Autodesk Inventor part; units mm, degrees
ref_plane "YZ Plane" through (0, 0, 0) normal (1, 0, 0) x (0, 1, 0)
ref_plane "XZ Plane" through (0, 0, 0) normal (0, 1, 0) x (-1, 0, 0)
ref_plane "XY Plane" through (0, 0, 0) normal (0, 0, 1) x (1, 0, 0)
sketch "Sketch1" plane through (0, 0, 0) normal (0, 0, 1) x (1, 0, 0)
  line L0 (-50, -180) -> (-450, -180)
  line L1 (-450, -180) -> (-450, 120)
  line L2 (-450, 120) -> (-50, 120)
  line L3 (-50, 120) -> (-50, -180)
  point P0 (0, 0)
  dimension "d0" = 50
  dimension "d1" = 300
  dimension "d2" = 400
  dimension "d3" = 120
extrude "Extrusion1" add sketch "Sketch1" along normal blind 120
sketch "Sketch2" plane through (-450, 120, 0) normal (0, 1, 0) x (1, 0, 0)
  line L0 (0, 0) -> (400, 0)
  line L1 (0, 0) -> (0, -120)
  line L2 (0, -120) -> (400, -120)
  line L3 (400, 0) -> (400, -120)
  line L4 (205, -30) -> (180, -30)
  line L5 (180, -30) -> (180, -20)
  line L6 (180, -20) -> (205, -20)
  line L7 (205, -20) -> (205, -30)
  dimension "d6" = 25
  dimension "d7" = 10
  dimension "d8" = 20
  dimension "d9" = 220
extrude "Extrusion2" add sketch "Sketch2" along normal blind 10 contours L4 L5 L6 L7
pattern_linear "Rectangular Pattern1" count 4 spacing 50 along (-1, 0, 0) of "Extrusion2"
sketch "Sketch3" plane through (-450, 120, 0) normal (0, 1, 0) x (1, 0, 0)
  line L0 (0, -120) -> (400, -120)
  line L1 (400, 0) -> (400, -120)
  line L2 (0, 0) -> (400, 0)
  line L3 (0, 0) -> (0, -120)
  line L4 (15, -65) -> (300, -65)
  line L5 (300, -65) -> (300, -105)
  line L6 (300, -105) -> (15, -105)
  line L7 (15, -105) -> (15, -65)
  line L8 (330, -65) -> (345, -65)
  line L9 (345, -65) -> (345, -105)
  line L10 (345, -105) -> (330, -105)
  line L11 (330, -105) -> (330, -65)
  line L12 (360, -65) -> (375, -65)
  line L13 (375, -65) -> (375, -105)
  line L14 (375, -105) -> (360, -105)
  line L15 (360, -105) -> (360, -65)
  point P0 (450, 0)
  dimension "d15" = 65
  dimension "d16" = 15
  dimension "d17" = 15
  dimension "d18" = 100
  dimension "d21" = 30
  dimension "d22" = 15
  dimension "d23" = 15
extrude "Extrusion3" cut sketch "Sketch3" against normal blind 5 contours L4 L5 L6 L7 | L8 L9 L10 L11 | L12 L13 L14 L15
chamfer "Chamfer1" distance 4 angle 45 3 edges at (-450, -30, 120) (-450, -30, 0) (-50, -30, 0)
sketch "Sketch4" plane through (-446, 120, 0) normal (0, 1, 0) x (1, 0, 0)
  line L0 (392, 0) -> (396, -4)
  line L1 (0, 0) -> (392, 0)
  line L2 (-4, -4) -> (0, 0)
  line L3 (-4, -4) -> (-4, -116)
  line L4 (0, -120) -> (-4, -116)
  line L5 (0, -120) -> (396, -120)
  line L6 (396, -4) -> (396, -120)
  line L7 (389.8859, -5.1039) -> (390.8961, -6.1141)
  line L8 (390.8961, -6.1141) -> (390.8961, -114.8961)
  line L9 (390.8961, -114.8961) -> (2.1141, -114.8961)
  line L10 (2.1141, -114.8961) -> (1.1039, -113.8859)
  line L11 (1.1039, -113.8859) -> (1.1039, -6.1141)
  line L12 (1.1039, -6.1141) -> (2.1141, -5.1039)
  line L13 (2.1141, -5.1039) -> (389.8859, -5.1039)
  point P0 (446, 0)
extrude "Extrusion4" add sketch "Sketch4" along normal blind 2
properties part number "AbstractBox"
The listing builds one solid part. Answer for the finished solid, in the listing's coordinates (mm). A direction names the side the tool comes from. Coordinates: 2 decimals unless noted, no trailing zeros. Order: outer loops, then holes, each group sorted by start corner. A loop starts at its lowest first (then second) coordinate and runs counter-clockwise, first axis right, second up. Notation, with made-up numbers: M 53,-34 L 98,-34 A5 ccw 98,-26 Z; hole C 33,-23.5 d11. An arc over 180 degrees is marked long. Answer as a JSON object with one key per item and string values. Group by question number.
1. A tool of negligible diameter and unlimited length cuts with its end or side. For faces 4 (the flat face through (-50, -31, 61)), 5 (the flat face through (-345, 125, 25)), from which of +Z, -Z, +X, -X, +Y, -Y can it reach the whole face along a straight path? Write none if from no direction.
2. Section B-B on x = -140 is taken. Write down the section's boundary in (y, z).
3. Section D-D on z = 79.5 is taken. Write down the section's boundary in (x, y).
4. Straight lines are drawn through the part: line 1 (Y direction, x = -404.5, z = 49); line 2 (Y direction, x = -237, z = 96.5). For each, find the intervals that lie inside material, in ascending order.
5. Section C-C on x = -334.5 is taken. Write down the section's boundary in (y, z), then the cut area to 3 significant figures.
6. Section A-A on z = 40.5 is taken. Write down the section's boundary in (x, y).
7. Flat-ended cylindrical pins translate along their axes: P1, Ø5, axis at x = -351.5, y = 125.5, coming from the -Z side; P2, Ø5, axis at x = -358.5, y = 126.5, coming from the +Z side; P3, Ø10, axis at x = -156.5, z = 26.5, coming from the +Y side. Find the tip coordinate at first contact, or state that the pin passes through.
8. Determine the mould class of faces 1 (the flat face through (-251, -31, 120)), 2 (the flat face through (-295, 125, 25)), 3 (the flat face through (-450, -31, 59)) for opening direction Z: released by +Z, released by -Z, zero draft, split by the parting line, or undercut.
Values follow:
{
 "1": {"face 4": "+Z, -Z, +X, +Y, -Y", "face 5": "+Y"},
 "2": {"outline": "M -180,0 L 122,0 L 122,5.1 L 120,5.1 L 120,114.9 L 122,114.9 L 122,120 L -180,120 Z"},
 "3": {"outline": "M -450,-180 L -50,-180 L -50,122 L -55.1,122 L -55.1,120 L -75,120 L -75,115 L -90,115 L -90,120 L -105,120 L -105,115 L -120,115 L -120,120 L -150,120 L -150,115 L -435,115 L -435,120 L -444.9,120 L -444.9,122 L -450,122 Z"},
 "4": {"line 1": "-180 to 120", "line 2": "-180 to 115"},
 "5": {"outline": "M -180,0 L 122,0 L 122,5.1 L 120,5.1 L 120,65 L 115,65 L 115,105 L 120,105 L 120,114.9 L 122,114.9 L 122,120 L -180,120 Z", "area": "35,800 mm2"},
 "6": {"outline": "M -450,-180 L -50,-180 L -50,122 L -55.1,122 L -55.1,120 L -444.9,120 L -444.9,122 L -450,122 Z"},
 "7": {"P1": "z = 20", "P2": "z = 30", "P3": "y = 120"},
 "8": {"face 1": "released by +Z", "face 2": "undercut", "face 3": "zero draft"}
}
